Design review of the part built by this model. Coordinates are the model's own, in mm. Face numbers are marked on the shaded views. A direction names the side the tool comes from. Round coordinates to 2 decimals unless told otherwise and drop trailing zeros. Order: outer loops, then holes, each group sorted by start corner. A loop starts at its lowest first (then second) coordinate and runs counter-clockwise, first axis right, second up.
from build123d import *

# Parameters (mm, degrees)
SKETCH1_W                       = 12.7
SKETCH1_H                       = 19.05
BOSS_EXTRUDE1_DEPTH             = 57.15
F_6_32_TAPPED_HOLE1_D           = 2.7051
F_6_32_TAPPED_HOLE1_DEPTH       = 12.7
F_6_32_TAPPED_HOLE1_CBORE_D     = 3.5052
F_6_32_TAPPED_HOLE1_CBORE_DEPTH = 10.795
F_6_32_TAPPED_HOLE1_TIP         = 0.81269403
CUT_EXTRUDE2_DEPTH              = 62.565534189
F_4_40_TAPPED_HOLE1_D           = 2.2606
CUT_EXTRUDE3_DEPTH              = 62.565534189


with BuildPart() as part:
    # Sketch1 → Boss-Extrude1 (new body)
    with BuildSketch(Plane(origin=(0, 0, 0), x_dir=(0, 0, -1), z_dir=(1, 0, 0))):
        with Locations((6.35, 9.525)):
            Rectangle(SKETCH1_W, SKETCH1_H)
    extrude(amount=-BOSS_EXTRUDE1_DEPTH)

    # #6-32 Tapped Hole1
    with Locations(Plane(origin=(23.287154444, 0, 3.188270264), x_dir=(1, 0, 0), z_dir=(0, -1, 0))):
        with Locations((-29.637154444, -9.538270264), (-74.087154444, -9.538270264)):
            CounterBoreHole(F_6_32_TAPPED_HOLE1_D / 2, F_6_32_TAPPED_HOLE1_CBORE_D / 2, F_6_32_TAPPED_HOLE1_CBORE_DEPTH, depth=F_6_32_TAPPED_HOLE1_DEPTH)
            with Locations((0, 0, -(F_6_32_TAPPED_HOLE1_DEPTH + F_6_32_TAPPED_HOLE1_TIP / 2))):  # 118° drill point
                Cone(0, F_6_32_TAPPED_HOLE1_D / 2, F_6_32_TAPPED_HOLE1_TIP, mode=Mode.SUBTRACT)

    # Sketch5 → Cut-Extrude2 (cut, through all)
    with BuildSketch(Plane(origin=(0, 0, -12.7), x_dir=(-1, 0, 0), z_dir=(0, 0, -1))):
        with BuildLine():
            Line((32.385, 19.05), (32.385, 13.97))
            ThreePointArc((32.385, 13.97), (26.035, 7.62), (19.685, 13.97))
            Line((19.685, 13.97), (19.685, 19.05))
            ThreePointArc((19.685, 19.05), (26.035, 25.4), (32.385, 19.05))
        make_face()
    extrude(amount=-CUT_EXTRUDE2_DEPTH, mode=Mode.SUBTRACT)

    # #4-40 Tapped Hole1 (through all)
    with Locations(Plane(origin=(0, 0, -12.7), x_dir=(-1, 0, 0), z_dir=(0, 0, -1))):
        with Locations((13.589, 13.97), (38.481, 13.97)):
            Hole(F_4_40_TAPPED_HOLE1_D / 2)

    # Sketch6 → Cut-Extrude3 (cut, through all)
    with BuildSketch(Plane(origin=(0, 0, -12.7), x_dir=(-1, 0, 0), z_dir=(0, 0, -1))):
        with BuildLine():
            Line((33.2105, 0), (42.9895, 0))
            Line((42.9895, 0), (42.9895, 0.127))
            ThreePointArc((42.9895, 0.127), (41.594596045, 3.494596045), (38.227, 4.8895))
            Line((38.227, 4.8895), (37.973, 4.8895))
            ThreePointArc((37.973, 4.8895), (34.605403955, 3.494596045), (33.2105, 0.127))
            Line((33.2105, 0.127), (33.2105, 0))
        make_face()
    extrude(amount=-CUT_EXTRUDE3_DEPTH, mode=Mode.SUBTRACT)


solid = part.part
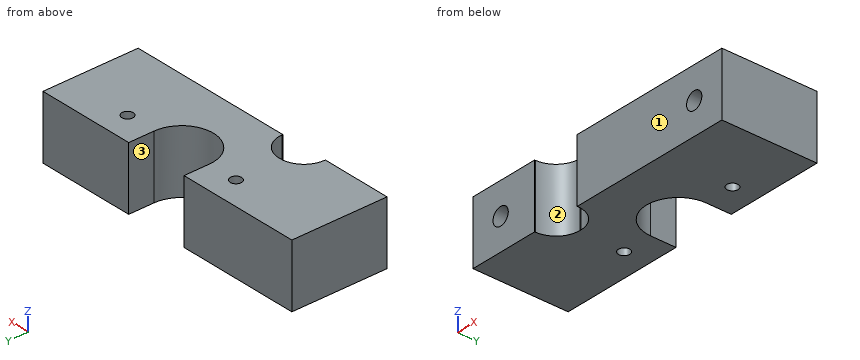
1) Take a section at C-C on y = 2.75. Give the boundary of the cut face in (x, z), plus the area to 3 significant figures.
Results:
outline: (-57.15, -12.7) - (-42.2, -12.7) - (-42.2, 0) - (-57.15, 0) - close; (-34, -12.7) - (0, -12.7) - (0, 0) - (-34, 0) - close; hole circle Ø3.51 at (-50.8, -6.35); hole circle Ø3.51 at (-6.35, -6.35)
area: 602 mm2
2) Clearance check with flat-ended pins moving along their axes: P1, Ø3, axis at x = -50.8, z = -6.35, coming from the -Y side (3 decimals); P2, Ø1, axis at x = -36, z = -6, coming from the -Y side; P3, Ø1.8, axis at x = -6.5, z = -6.5, coming from the -Y side; P4, Ø1.8, axis at x = -13.589, y = 13.97, coming from the +Z side. State where each tip first meets the part, or that it passes through.
Results:
P1: stops at y = 10.795
P2: stops at y = 4.2
P3: stops at y = 12.84
P4: passes through
3) Take a section at B-B on z = -11. State how many separate pieces and enclosed holes the cut face has, plus the area to 3 significant figures.
Results:
separate pieces: 1
enclosed holes: 2
area: 915 mm2
4) Take a section at A-A on y = 16.25. Give the boundary of the cut face in (x, z) (3 decimals).
Results:
outline: (-57.15, -12.7) - (-32.385, -12.7) - (-32.385, 0) - (-57.15, 0) - close; (-19.685, -12.7) - (0, -12.7) - (0, 0) - (-19.685, 0) - close
5) To check wall thickness, follow line 1 along X through (y, z) = (17.75, -7) (3 decimals); line 2 along Z through (x, y) = (-50.8, 11.2); line 3 along Z through (x, y) = (-6.35, 5). State the ranges of each line that lie inside material, in increasing order.
Results:
line 1: x = -57.15 to -32.385, -19.685 to 0
line 2: z = -12.7 to -7.7, -5 to 0
line 3: z = -12.7 to -8.1, -4.6 to 0
6) For the marked faces 1, 2 and 3, list the 3-axis set-ups (+Z, -Z, +X, -X, +Y, -Y) from which the entire face can be reached by the end or side of a thin tool; tool diameter is ignored.
Results:
face 1: +Z, -Z, +X, -X, -Y
face 2: +Z, -Z, -Y
face 3: +Z, -Z, +Y
7) Take a section at D-D on y = 6.5. Give the boundary of the cut face in (x, z), plus the area to 3 significant figures.
Results:
outline: (-57.15, -12.7) - (0, -12.7) - (0, 0) - (-57.15, 0) - close; hole circle Ø3.51 at (-50.8, -6.35); hole circle Ø3.51 at (-6.35, -6.35)
area: 707 mm2
